Can you work these out from the drawing? Everything is in mm from the part's minimum corner. A direction names the side the tool comes from. Give positions to 0.01 mm unless a question says otherwise; leave off trailing zeros. Order: outer loops, then holes, each group sorted by start corner. A loop starts at its lowest first (then second) coordinate and runs counter-clockwise, first axis right, second up. Notation, with made-up numbers: M 75,-36.5 L 121,-36.5 A23 ccw 121,-21.5 Z; hole C 3.5,40.5 d4. An arc over 180 degrees is marked long. Answer as a JSON object with one key per item and string values.
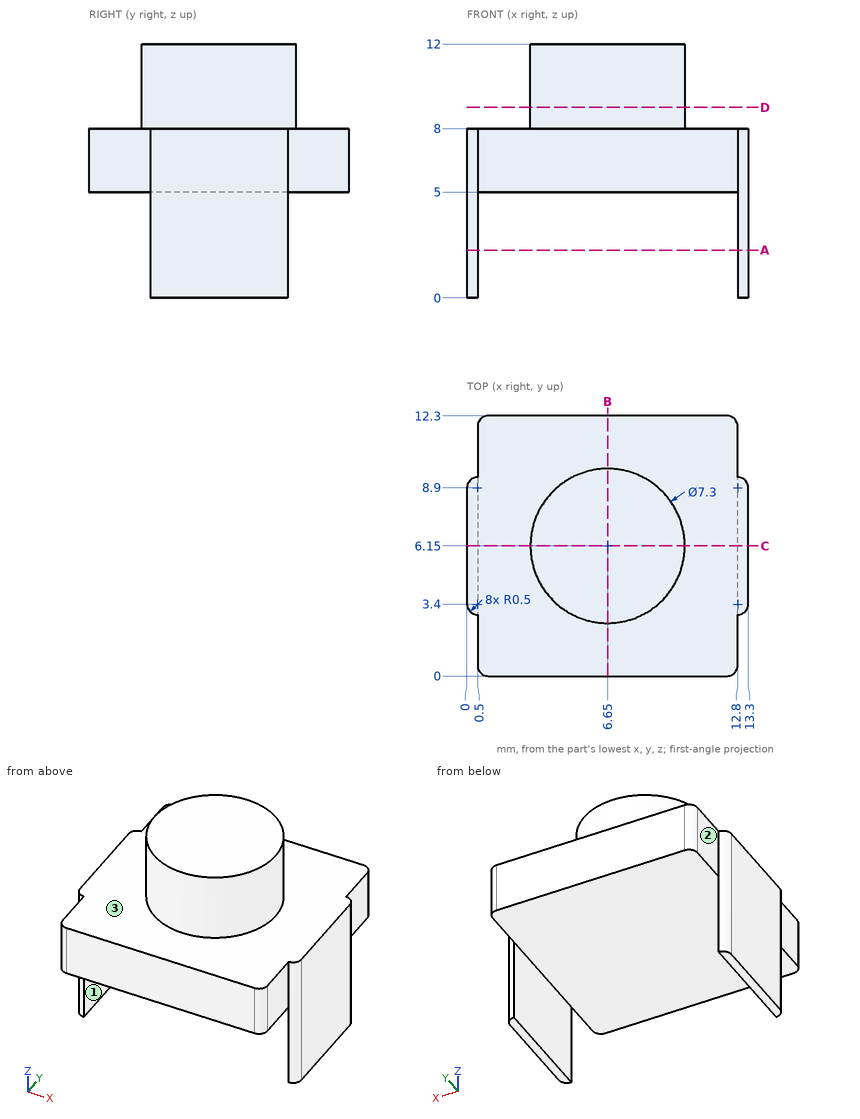
1) I want a section at B-B on x = 6.65. Write out the boundary of the cut face in (y, z), and give its area (3 significant figures).
Results found:
{"outline": "M 0,5 L 12.3,5 L 12.3,8 L 9.8,8 L 9.8,12 L 2.5,12 L 2.5,8 L 0,8 Z", "area": "66.1 mm²"}
2) I need wall thicknesses on L1, parallel to X at y = 6.25, z = 1.5; L2, parallel to Z at x = 6.25, y = 8.75; L3, parallel to X at y = 11.5, z = 5.5. Which ranges of each line are inside material? Lowest first, please.
Results found:
{"L1": "x = 0 to 0.5, 12.8 to 13.3", "L2": "z = 5 to 12", "L3": "x = 0.5 to 12.8"}
3) For the marked faces 1, 2 and 3, which set-ups out of +Z, -Z, +X, -X, +Y, -Y let a thin tool reach every point of the face, with its end or its side?
Results found:
{"face 1": "-Z, +Y, -Y", "face 2": "+Z, -Z, -X, +Y", "face 3": "+Z"}
4) I want a section at A-A on z = 2.25. Write out the boundary of the cut face in (x, y).
Results found:
{"outline": "M 0,3.4 A0.5 ccw 0.5,2.9 L 0.5,9.4 A0.5 ccw 0,8.9 Z; M 12.8,2.9 A0.5 ccw 13.3,3.4 L 13.3,8.9 A0.5 ccw 12.8,9.4 Z"}
5) I want a section at D-D on z = 9. Write out the boundary of the cut face in (x, y), and give its area (3 significant figures).
Results found:
{"outline": "C 6.65,6.15 d7.3", "area": "41.9 mm²"}
6) I'm going to push flat-ended pins straight in: pin 1 Ø1 at (y, z) = (3, 5.5) entering from +X; pin 2 Ø6 at (x, y) = (7, 7) entering from -Z; pin 3 Ø1.2 at (y, z) = (10.5, 6) entering from +X; pin 4 Ø1.9 at (y, z) = (11, 6) entering from -X. Where does each tip first touch, or does it pass through?
Results found:
{"pin 1": "stops at x = 13.3", "pin 2": "stops at z = 5", "pin 3": "stops at x = 12.8", "pin 4": "stops at x = 0.5"}
7) I want a section at C-C on y = 6.15. Write out the boundary of the cut face in (x, z), and give its area (3 significant figures).
Results found:
{"outline": "M 0,0 L 0.5,0 L 0.5,5 L 12.8,5 L 12.8,0 L 13.3,0 L 13.3,8 L 10.3,8 L 10.3,12 L 3,12 L 3,8 L 0,8 Z", "area": "74.1 mm²"}
